Autodesk Fusion 360 part; units mm, degrees
sketch "Schizzo2" plane through (0, 0, 0) normal (0, 1, 0) x (1, 0, 0)
  line L0 (0, 0) -> (2, 0)
  line L1 (2, 0) -> (2, -30)
  line L2 (2, -30) -> (0, -30)
  line L3 (0, -30) -> (0, 0)
  line L4 (2, -30) -> (5, -30)
  line L5 (5, -30) -> (5, -15)
  line L6 (5, -15) -> (2, -15)
  line L7 (2, -15) -> (2, -30)
  line L8 (5, -30) -> (10, -30)
  line L9 (10, -30) -> (10, 0)
  line L10 (10, 0) -> (5, 0)
  line L11 (5, 0) -> (5, -30)
  dimension "d1" = 2
  dimension "d2" = 30
  dimension "d3" = 3
  dimension "d4" = 30
  dimension "d5" = 5
  dimension "d44" = 15
extrude "Estrusione1" add sketch "Schizzo2" along normal blind 200
sketch "Schizzo3" plane through (10, 0, 0) normal (1, 0, 0) x (0, 1, 0)
  line L0 (0, 30) -> (0, 0)
  line L1 (0, 0) -> (200, 0)
  line L2 (200, 0) -> (200, 30)
  line L3 (200, 30) -> (0, 30)
  line L4 (0, 30) -> (10, 30)
  circle A0 centre (10, 4) radius 3.5
  line L5 (6, 0) -> (6.5245, 4.413)
  line L6 (14, 0) -> (13.4755, 4.413)
  line L7 (6, 0) -> (14, 0)
  dimension "d8" = 7
extrude "Estrusione2" add sketch "Schizzo3" along normal blind 13 contours L1 A0 L5 L6 L7 | A0
sketch "Schizzo4" plane through (23, 0, 0) normal (1, 0, 0) x (0, 1, 0)
  line L0 (3, 0) -> (17, 0)
  line L1 (17, 0) -> (17, 10)
  line L2 (17, 10) -> (3, 10)
  line L3 (3, 10) -> (3, 0)
extrude "Estrusione4" add sketch "Schizzo4" along normal blind 5
fillet "Raccordo3" radius 1.5 8 edges at (23, 10, 10) (25.5, 17, 10) (28, 10, 10) (25.5, 3, 10) (28, 3, 5) (23, 3, 5) (28, 17, 5) (23, 17, 5)
sketch "Schizzo5" plane through (10, 0, 0) normal (1, 0, 0) x (0, 1, 0)
  line L0 (13.4755, 4.413) -> (14, 0)
  line L1 (14, 0) -> (200, 0)
  line L2 (200, 0) -> (200, 30)
  line L3 (200, 30) -> (0, 30)
  line L4 (0, 30) -> (0, 0)
  line L5 (0, 0) -> (6, 0)
  line L6 (6, 0) -> (6.5245, 4.413)
  arc A0 (13.4755, 4.413) -> (6.5245, 4.413) centre (10, 4) ccw
sketch "Schizzo6" plane through (10, 0, 0) normal (1, 0, 0) x (0, 1, 0)
  line L0 (70, 0) -> (70, 4)
  line L1 (70, 0) -> (90, 0)
  line L2 (90, 0) -> (106, 0)
  line L3 (106, 0) -> (111, 0)
  line L4 (111, 0) -> (111, 4)
  line L5 (90, 0) -> (90, 4)
  line L6 (106, 0) -> (106, 4)
  line L7 (111, 4) -> (106, 4)
  line L8 (90, 4) -> (70, 4)
  dimension "d22" = 20
  dimension "d23" = 16
  dimension "d24" = 5
extrude "Estrusione5" add sketch "Schizzo6" along normal blind 9
sketch "Schizzo7" plane through (19, 0, 0) normal (1, 0, 0) x (0, 1, 0)
  line L0 (70, 0) -> (90, 0)
  line L1 (90, 0) -> (90, 4)
  line L2 (90, 4) -> (70, 4)
  line L3 (70, 4) -> (70, 0)
  line L4 (70, 0) -> (90, 0)
  line L5 (90, 0) -> (90, 7)
  line L6 (90, 7) -> (70, 7)
  line L7 (70, 7) -> (70, 0)
  line L8 (106, 0) -> (111, 0)
  line L9 (111, 0) -> (111, 7)
  line L10 (111, 7) -> (106, 7)
  line L11 (106, 7) -> (106, 0)
extrude "Estrusione6" add sketch "Schizzo7" along normal blind 3
fillet "Raccordo4" radius 1 12 edges at (19, 108.5, 7) (22, 108.5, 7) (22, 80, 7) (19, 80, 7) (20.5, 90, 7) (20.5, 106, 7) (20.5, 111, 7) (22, 106, 3.5) (22, 111, 3.5) (22, 90, 3.5) (20.5, 70, 7) (22, 70, 3.5)
sketch "Schizzo8" plane through (10, 0, 0) normal (1, 0, 0) x (0, 1, 0)
  line L0 (150, 0) -> (150, 10)
  line L1 (150, 0) -> (170, 0)
  line L2 (170, 0) -> (175, 5)
  line L3 (145, 5) -> (150, 0)
  line L4 (145, 5) -> (143, 5)
  line L5 (148, 0) -> (150, 0)
  line L6 (175, 5) -> (177, 5)
  line L7 (170, 0) -> (172, 0)
  line L8 (143, 5) -> (144, 0)
  line L9 (144, 0) -> (148, 0)
  line L10 (177, 5) -> (176, 0)
  line L11 (176, 0) -> (172, 0)
  dimension "d31" = 20
extrude "Estrusione8" add sketch "Schizzo8" along normal blind 10
sketch "Schizzo9" plane through (20, 0, 0) normal (1, 0, 0) x (0, 1, 0)
  line L0 (170, 0) -> (176, 0)
  line L1 (176, 0) -> (177, 5)
  line L2 (177, 5) -> (175, 5)
  line L3 (175, 5) -> (170, 0)
  line L4 (143, 5) -> (143, 6)
  line L5 (143, 6) -> (145, 6)
  line L6 (145, 6) -> (150, 1)
  line L7 (150, 1) -> (150, 0)
  line L8 (143, 5) -> (144, 0)
  line L9 (144, 0) -> (150, 0)
  line L10 (170, 0) -> (170, 1)
  line L11 (170, 1) -> (175, 6)
  line L12 (175, 6) -> (177, 6)
  line L13 (177, 6) -> (177, 5)
  line L14 (176, 0) -> (177, 5)
  line L15 (170, 0) -> (176, 0)
extrude "Estrusione9" add sketch "Schizzo9" along normal blind 3
fillet "Raccordo5" radius 1 4 edges at (23, 144, 6) (23, 147.5, 3.5) (23, 176, 6) (23, 172.5, 3.5)
sketch "Schizzo10" plane through (0, 200, 0) normal (0, 1, 0) x (-1, 0, 0)
  line L0 (0, 30) -> (-10, 30)
  line L1 (-10, 30) -> (-10, 0)
  line L2 (-10, 0) -> (-5, 0)
  line L3 (-5, 0) -> (-5, 15)
  line L4 (-5, 15) -> (-2, 15)
  line L5 (-2, 15) -> (-2, 0)
  line L6 (-2, 0) -> (0, 0)
  line L7 (0, 0) -> (0, 30)
  line L8 (-12, 31) -> (4, 31)
  line L9 (4, 31) -> (4, -5)
  line L10 (4, -5) -> (-12, -5)
  line L11 (-12, -5) -> (-12, 31)
extrude "Estrusione10" cut sketch "Schizzo10" against normal blind 23 contours L0 L1 L2 L3 L4 L5 L6 L7 | L8 L9 L10 L11
sketch "Schizzo11" plane through (0, 0, 0) normal (0, -1, 0) x (1, 0, 0)
  line L0 (10, 30) -> (0, 30)
  line L1 (0, 30) -> (0, 0)
  line L2 (0, 0) -> (2, 0)
  line L3 (2, 0) -> (2, 15)
  line L4 (2, 15) -> (5, 15)
  line L5 (5, 15) -> (5, 0)
  line L6 (5, 0) -> (10, 0)
  line L7 (10, 0) -> (10, 30)
  line L8 (-2, 31) -> (12, 31)
  line L9 (12, 31) -> (12, -1)
  line L10 (12, -1) -> (-2, -1)
  line L11 (-2, -1) -> (-2, 31)
extrude "Estrusione11" cut sketch "Schizzo11" against normal blind 6 contours L0 L1 L2 L3 L4 L5 L6 L7
sketch "Schizzo12" plane through (0, 6, 0) normal (0, -1, 0) x (1, 0, 0)
  line L0 (10, 0) -> (10, 30)
  line L1 (10, 30) -> (0, 30)
  line L2 (0, 30) -> (0, 0)
  line L3 (0, 0) -> (2, 0)
  line L4 (2, 0) -> (2, 15)
  line L5 (2, 15) -> (5, 15)
  line L6 (5, 15) -> (5, 0)
  line L7 (5, 0) -> (10, 0)
  line L8 (-2, 31) -> (11, 31)
  line L9 (11, 31) -> (11, 18)
  line L10 (11, 18) -> (-2, 18)
  line L11 (-2, 18) -> (-2, 31)
  dimension "d45" = 13
extrude "Estrusione12" cut sketch "Schizzo12" against normal blind 175 contours L0 L1 L2 L10
sketch "Schizzo13" plane through (0, 0, 0) normal (-1, 0, 0) x (0, -1, 0)
  line L0 (-6, 18) -> (-177, 18)
  line L1 (-177, 18) -> (-177, 0)
  line L2 (-177, 0) -> (-6, 0)
  line L3 (-6, 0) -> (-6, 18)
  line L4 (-177, 18) -> (-6, 18)
  line L5 (-6, 18) -> (-6, 0)
  line L6 (-6, 0) -> (-177, 0)
  line L7 (-177, 0) -> (-177, 18)
sketch "Schizzo14" plane through (10, 0, 0) normal (1, 0, 0) x (0, 1, 0)
  line L0 (56, 0) -> (58, 0)
  line L1 (58, 0) -> (58, 6)
  line L2 (58, 6) -> (56, 6)
  line L3 (56, 6) -> (56, 0)
  line L4 (70, 6) -> (70, 0)
  dimension "d48" = 12
  dimension "d49" = 2
  dimension "d50" = 6
extrude "Estrusione13" add sketch "Schizzo14" along normal blind 14
For this review, take the finished solid that the model builds, in its own axes (mm). A direction names the side the tool comes from. Give positions to 0.01 mm unless a question says otherwise; leave off trailing zeros. Loops run counter-clockwise (first coordinate to the right, second up) from the corner with the lowest first, then second, coordinate; pieces in that order, holes last. Notation, with made-up numbers: M 0,86.5 L 51,86.5 A18 ccw 51,90.5 Z; hole C 67,72 d8. An arc over 180 degrees is marked long. One line per item, written item: value. Start each with the question number.
Q1. Add section A-A (x = 16). Give the boundary of the cut face in (y, z).
Q2. For L1, parallel to X at y = 163.5, z = 14; L2, parallel to Y at x = 18.5, z = 2; L3, parallel to Y at x = 19.5, z = 2.5, list the stretches that pass through material, from the lowest coordinate up.
Q3. Add section D-D (x = 6.5). Give the boundary of the cut face in (y, z), and give its area (3 significant figures).
Q4. Clearance check with flat-ended pins moving along their axes: pin 1 Ø3.5 at (y, z) = (109, 3.5) entering from +X; pin 2 Ø3 at (x, y) = (20, 111.5) entering from +Z; pin 3 Ø6.5 at (x, z) = (14.5, 4) entering from -Y. State where each tip first meets the part, or that it passes through.
Q5. Add section B-B (z = 12.25). Give the boundary of the cut face in (x, y), and give its area (3 significant figures).
Q6. Machinability: for faces 4 (the face through (23, 146, 2)), 5 (the face through (15, 172, 2)), 6 (the face through (21, 172, 3)), 7 (the face through (22, 80, 3)), which of the approach directions +Z, -Z, +X, -X, +Y, -Y give a long, thin tool a straight path to every point of the face, cutting with its end or side? Answer none if there is none.
Q7. Add section C-C (y = 95.5). Give the boundary of the cut face in (x, z).
Q8. Draft analysis for pull direction Y (two halves, no side actions). For faces 1 (the face through (15, 70, 2)), 2 (the face through (15, 106, 2)), 3 (the face through (23, 174, 2)), state which applies: released by +Y, released by -Y, zero draft, split by the parting line, or undercut.
Reply:
1. outline: M 6,0 L 14,0 L 13.48,4.41 A3.5 ccw 6.52,4.41 Z; M 56,0 L 58,0 L 58,6 L 56,6 Z; M 70,0 L 90,0 L 90,4 L 70,4 Z; M 106,0 L 111,0 L 111,4 L 106,4 Z; M 143,5 L 144,0 L 150,0 L 145,5 Z; M 170,0 L 176,0 L 177,5 L 175,5 Z
2. L1: 0 to 2, 5 to 10
2. L2: 6.24 to 13.76, 56 to 58, 70 to 90, 106 to 111, 143.6 to 148, 172 to 176.4
2. L3: 6.3 to 13.7, 56 to 58, 70 to 90, 106 to 111, 143.5 to 147.5, 172.5 to 176.5
3. outline: M 6,0 L 177,0 L 177,18 L 6,18 Z
3. area: 3,080 mm²
4. pin 1: x = 22
4. pin 2: z = 7
4. pin 3: y = 6.09
5. outline: M 0,6 L 2,6 L 2,177 L 0,177 Z; M 5,6 L 10,6 L 10,177 L 5,177 Z
5. area: 1,200 mm²
6. face 4: +Z, -Z, +X, +Y
6. face 5: +Z
6. face 6: +Z, +X
6. face 7: +Z, -Z, +X
7. outline: M 0,0 L 2,0 L 2,15 L 5,15 L 5,0 L 10,0 L 10,18 L 0,18 Z
8. face 1: undercut
8. face 2: undercut
8. face 3: zero draft
